from build123d import *

# Parameters (mm, degrees)
SKETCH1_R            = 30
BOSS_EXTRUDE8_DEPTH  = 43.19
SKETCH1_9_R          = 32.5
SKETCH1_9_R_2        = 30
BOSS_EXTRUDE10_DEPTH = 5
SKETCH2_R            = 8
SKETCH2_R_2          = 6
CUT_EXTRUDE1_DEPTH   = 2
SKETCH3_R            = 15
SKETCH3_R_2          = 12.5
CUT_EXTRUDE2_DEPTH   = 3


with BuildPart() as part:
    # Sketch1 → Boss-Extrude8 (new body)
    with BuildSketch(Plane(origin=(0, 0, 0), x_dir=(1, 0, 0), z_dir=(0, 1, 0))):
        Circle(SKETCH1_R)
    extrude(amount=-BOSS_EXTRUDE8_DEPTH)

    # Sketch1<9> → Boss-Extrude10 (add)
    with BuildSketch(Plane(origin=(0, 0, 0), x_dir=(1, 0, 0), z_dir=(0, 1, 0))):
        Circle(SKETCH1_9_R)
        Circle(SKETCH1_9_R_2, mode=Mode.SUBTRACT)
    extrude(amount=-BOSS_EXTRUDE10_DEPTH)

    # Sketch2 → Cut-Extrude1 (cut)
    with BuildSketch(Plane.XZ.offset(43.19)):
        Circle(SKETCH2_R)
        Circle(SKETCH2_R_2, mode=Mode.SUBTRACT)
    extrude(amount=-CUT_EXTRUDE1_DEPTH, mode=Mode.SUBTRACT)

    # Sketch3 → Cut-Extrude2 (cut)
    with BuildSketch(Plane(origin=(0, 0, 0), x_dir=(1, 0, 0), z_dir=(0, 1, 0))):
        Circle(SKETCH3_R)
        Circle(SKETCH3_R_2, mode=Mode.SUBTRACT)
    extrude(amount=-CUT_EXTRUDE2_DEPTH, mode=Mode.SUBTRACT)


solid = part.part
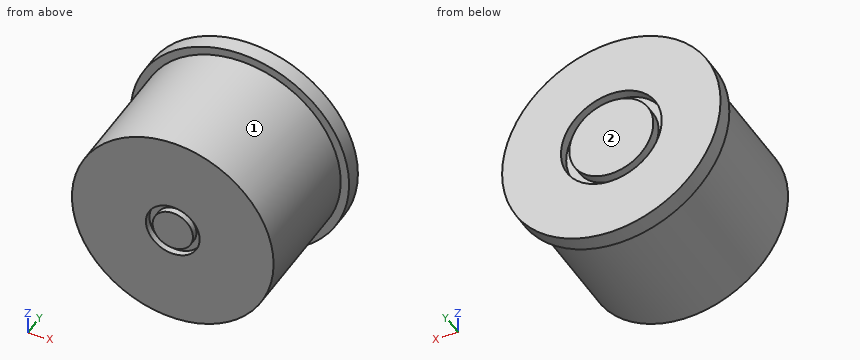
Could you check a few things on this model? Use its own coordinates, in mm. Face numbers are marked on the shaded views. A direction names the side the tool comes from. Give positions to 0.01 mm unless a question says otherwise; leave off trailing zeros. Order: outer loops, then holes, each group sorted by start corner. A loop starts at its lowest first (then second) coordinate and runs counter-clockwise, first axis right, second up. Notation, with made-up numbers: (48, 27.25) -> (85, 27.25) arc R27 cw to (85, 56.25) -> close; hole circle Ø7 at (73, -9). An arc over 180 degrees is marked (long way). Answer in a Markdown table with one row per item. Add a question column.
Item 1: Imagine slicing it at C-C (y = -19.5). List the corners of the cut face in (x, z) for me, and give its area (3 significant figures).
Item 2: Please list where these lines run through material, in increasing order: probe 1 along Z at (x, y) = (0, -1); probe 2 along Z at (x, y) = (0, -42.2).
Item 3: Imagine slicing it at A-A (z = 0). List the corners of the cut face in (x, y) for me.
Item 4: Imagine slicing it at D-D (z = 20). List the corners of the cut face in (x, y) for me, and give its area (3 significant figures).
Item 5: I'm going to push flat-ended pins straight in: P1, Ø2, axis at y = -29.5, z = 9, coming from the +X side; P2, Ø6, axis at x = 4.5, y = -13.5, coming from the +Z side; P3, Ø12, axis at y = -14, z = 13.5, coming from the -X side; P4, Ø9, axis at x = -2, z = 3, coming from the +Y side. Where does each tip first touch, or does it pass through?
Item 6: Imagine slicing it at B-B (x = 0). List the corners of the cut face in (y, z) for me.
Item 7: For the marked faces 1 and 2, which set-ups out of +Z, -Z, +X, -X, +Y, -Y let a thin tool reach every point of the face, with its end or its side?
Result:
| question | item | result |
|---|---|---|
| 1 | outline | circle Ø60 at (0, 0) |
| 1 | area | 2,830 mm2 |
| 2 | probe 1 | -32.5 to -15, -12.5 to 12.5, 15 to 32.5 |
| 2 | probe 2 | -30 to -8, -6 to 6, 8 to 30 |
| 3 | outline | (-32.5, -5) -> (-30, -5) -> (-30, -43.19) -> (-8, -43.19) -> (-8, -41.19) -> (-6, -41.19) -> (-6, -43.19) -> (6, -43.19) -> (6, -41.19) -> (8, -41.19) -> (8, -43.19) -> (30, -43.19) -> (30, -5) -> (32.5, -5) -> (32.5, 0) -> (15, 0) -> (15, -3) -> (12.5, -3) -> (12.5, 0) -> (-12.5, 0) -> (-12.5, -3) -> (-15, -3) -> (-15, 0) -> (-32.5, 0) -> close |
| 4 | outline | (-25.62, -5) -> (-22.36, -5) -> (-22.36, -43.19) -> (22.36, -43.19) -> (22.36, -5) -> (25.62, -5) -> (25.62, 0) -> (-25.62, 0) -> close |
| 4 | area | 1,960 mm2 |
| 5 | P1 | x = 28.91 |
| 5 | P2 | z = 29.96 |
| 5 | P3 | x = -29.05 |
| 5 | P4 | y = 0 |
| 6 | outline | (-43.19, -30) -> (-5, -30) -> (-5, -32.5) -> (0, -32.5) -> (0, -15) -> (-3, -15) -> (-3, -12.5) -> (0, -12.5) -> (0, 12.5) -> (-3, 12.5) -> (-3, 15) -> (0, 15) -> (0, 32.5) -> (-5, 32.5) -> (-5, 30) -> (-43.19, 30) -> (-43.19, 8) -> (-41.19, 8) -> (-41.19, 6) -> (-43.19, 6) -> (-43.19, -6) -> (-41.19, -6) -> (-41.19, -8) -> (-43.19, -8) -> close |
| 7 | face 1 | -Y |
| 7 | face 2 | +Z, -Z, +X, -X, +Y |
